from build123d import *

# Parameters (mm, degrees)
SALIENTE_EXTRUIR1_DEPTH = 6.35
CROQUIS3_R              = 1.5
CROQUIS3_R_2            = 2
CORTAR_EXTRUIR2_DEPTH   = 7.35
CORTAR_EXTRUIR3_DEPTH   = 56
REDONDEO2_R             = 1.5
CROQUIS5_R              = 2
CORTAR_EXTRUIR5_DEPTH   = 7.3500001
CROQUIS7_R              = 3.75
CORTAR_EXTRUIR6_DEPTH   = 3.5
CROQUIS8_R              = 1.5
CORTAR_EXTRUIR7_DEPTH   = 7.3500001


with BuildPart() as part:
    # Croquis1 → Saliente-Extruir1 (new body)
    with BuildSketch(Plane.XY):
        with BuildLine():
            Line((92.5, 23), (50, 23))
            Line((50, 23), (-1.986430717, 16.883545037))
            ThreePointArc((-1.986430717, 16.883545037), (-17, 0), (-1.986430717, -16.883545037))
            Line((-1.986430717, -16.883545037), (50, -23))
            Line((50, -23), (92.5, -23))
            Line((92.5, -23), (110, -18))
            Line((110, -18), (160, -18))
            Line((160, -18), (177.5, -23))
            Line((177.5, -23), (220, -23))
            Line((220, -23), (271.986430717, -16.883545037))
            ThreePointArc((271.986430717, -16.883545037), (287, 0), (271.986430717, 16.883545037))
            Line((271.986430717, 16.883545037), (220, 23))
            Line((220, 23), (177.5, 23))
            Line((177.5, 23), (160, 18))
            Line((160, 18), (110, 18))
            Line((110, 18), (92.5, 23))
        make_face()
    extrude(amount=SALIENTE_EXTRUIR1_DEPTH)

    # Croquis3 → Cortar-Extruir2 (cut, through all)
    with BuildSketch(Plane.XY.offset(6.35)):
        with Locations((52, 11)):
            Circle(CROQUIS3_R)
        with Locations((52, -11)):
            Circle(CROQUIS3_R)
        with Locations((218, -11)):
            Circle(CROQUIS3_R)
        with Locations((218, 11)):
            Circle(CROQUIS3_R)
        with Locations((135, 0)):
            Circle(CROQUIS3_R_2)
    extrude(amount=-CORTAR_EXTRUIR2_DEPTH, mode=Mode.SUBTRACT)

    # Croquis2 → Cortar-Extruir3 (cut)
    with BuildSketch(Plane.XY.offset(6.35)):
        with BuildLine():
            ThreePointArc((-3.348857081, 7.8125), (-4.530250685, 7.19213659), (-5.6, 6.394528911))
            Line((-5.6, 6.394528911), (-5.6, -6.394528911))
            ThreePointArc((-5.6, -6.394528911), (-4.530250685, -7.19213659), (-3.348857081, -7.8125))
            ThreePointArc((-3.348857081, -7.8125), (0, -14), (3.348857081, -7.8125))
            ThreePointArc((3.348857081, -7.8125), (4.530250685, -7.19213659), (5.6, -6.394528911))
            Line((5.6, -6.394528911), (5.6, 6.394528911))
            ThreePointArc((5.6, 6.394528911), (4.530250685, 7.19213659), (3.348857081, 7.8125))
            ThreePointArc((3.348857081, 7.8125), (0, 14), (-3.348857081, 7.8125))
        make_face()
    extrude(amount=-CORTAR_EXTRUIR3_DEPTH, mode=Mode.SUBTRACT)

    # Redondeo2
    redondeo2_edges = [part.edges().sort_by_distance(p)[0] for p in [
        (-3.348857081, 7.8125, 3.175),
        (3.348857081, 7.8125, 3.175),
        (3.348857081, -7.8125, 3.175),
        (-3.348857081, -7.8125, 3.175),
    ]]
    fillet(redondeo2_edges, radius=REDONDEO2_R)

    # Croquis5 → Cortar-Extruir5 (cut, through all)
    with BuildSketch(Plane.XY.offset(6.35)):
        with Locations((25, 15.263279564)):
            Circle(CROQUIS5_R)
        with Locations((25, -15.263279564)):
            Circle(CROQUIS5_R)
        with Locations((102.242759853, 15.263279564)):
            Circle(CROQUIS5_R)
        with Locations((102.242759853, -15.263279564)):
            Circle(CROQUIS5_R)
        with Locations((167.757240147, -15.263279564)):
            Circle(CROQUIS5_R)
        with Locations((167.757240147, 15.263279564)):
            Circle(CROQUIS5_R)
        with Locations((245, 15.263279564)):
            Circle(CROQUIS5_R)
        with Locations((245, -15.263279564)):
            Circle(CROQUIS5_R)
    extrude(amount=-CORTAR_EXTRUIR5_DEPTH, mode=Mode.SUBTRACT)

    # Croquis7 → Cortar-Extruir6 (cut)
    with BuildSketch(Plane.XY.offset(6.35)):
        with Locations((25, 15.263279564)):
            Circle(CROQUIS7_R)
        with Locations((25, -15.263279564)):
            Circle(CROQUIS7_R)
        with Locations((245, 15.263279564)):
            Circle(CROQUIS7_R)
        with Locations((245, -15.263279564)):
            Circle(CROQUIS7_R)
        with Locations((102.242759853, 15.263279564)):
            Circle(CROQUIS7_R)
        with Locations((102.242759853, -15.263279564)):
            Circle(CROQUIS7_R)
        with Locations((167.757240147, -15.263279564)):
            Circle(CROQUIS7_R)
        with Locations((167.757240147, 15.263279564)):
            Circle(CROQUIS7_R)
    extrude(amount=-CORTAR_EXTRUIR6_DEPTH, mode=Mode.SUBTRACT)

    # Croquis8 → Cortar-Extruir7 (cut, through all)
    with BuildSketch(Plane.XY.offset(6.35)):
        with Locations((248, 0)):
            Circle(CROQUIS8_R)
        with Locations((250.397856468, 9.987790994)):
            Circle(CROQUIS8_R)
        with Locations((258.509333353, 9.641814145)):
            Circle(CROQUIS8_R)
        with Locations((258.509333353, -9.641814145)):
            Circle(CROQUIS8_R)
        with Locations((250.397856468, -9.987790994)):
            Circle(CROQUIS8_R)
    extrude(amount=-CORTAR_EXTRUIR7_DEPTH, mode=Mode.SUBTRACT)


solid = part.part
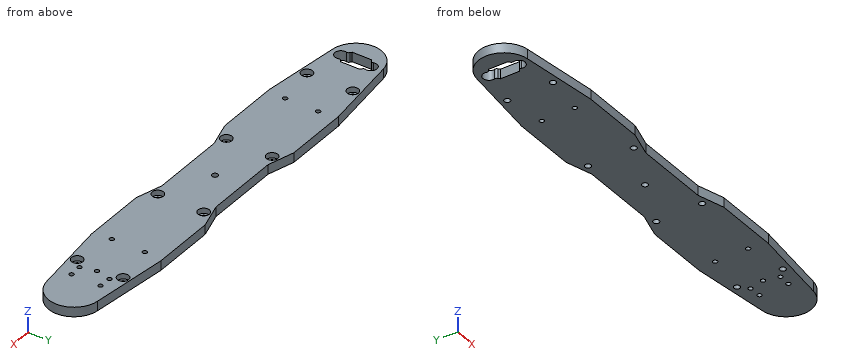
Build history of the part. All positions in model axes, mm. Coordinates: 2 decimals unless noted, no trailing zeros. Write each loop counter-clockwise with the first axis right and the second up, starting at its lowest first coordinate (ties: lowest second). Pieces come first, ordered by that corner, then holes.
(1) Cut at A-A on z = 4.75. State how many separate pieces and enclosed holes the cut face has, and give its area (3 significant figures).
(2) Drill centre lines: line 1 (Y direction, x = 218, z = 3.25); line 2 (X direction, y = 10.5, z = 2.25); line 3 (X direction, y = 10, z = 4.5). Where is each one in solid material? Low to high.
(3) Cut at B-B on x = 124. List the corners of the cut face in (y, z), and give its area (3 significant figures).
(4) Cut at C-C on x = 15. List the corners of the cut face in (y, z), and give its area (3 significant figures).
(5) Pin check, flat tips, straight feed: pin 1 Ø1.5 at (y, z) = (7.5, 1.5) entering from -X; pin 2 Ø6 at (x, y) = (245, -15.26) entering from +Z. Stop position of each tip, or through.
Working result:
1. separate pieces: 1
1. enclosed holes: 19
1. area: 11,400 mm2
2. line 1: y = -23 to -12.5, -9.5 to 9.5, 12.5 to 23
2. line 2: x = -13.37 to -3.97, 3.97 to 50.59, 53.41 to 216.59, 219.41 to 248.99, 251.81 to 257.28, 259.74 to 283.37
2. line 3: x = -13.75 to -4, 4 to 50.88, 53.12 to 216.88, 219.12 to 248.9, 251.9 to 257.05, 259.97 to 283.75
3. outline: (-18, 0) - (18, 0) - (18, 6.35) - (-18, 6.35) - close
3. area: 229 mm2
4. outline: (-18.88, 0) - (18.88, 0) - (18.88, 6.35) - (-18.88, 6.35) - close
4. area: 240 mm2
5. pin 1: stops at x = -15.6
5. pin 2: stops at z = 2.85
